Read the model definition and answer for the solid it produces. Units are mm, in the model's axes. A direction names the side the tool comes from. Give positions to 0.01 mm unless a question says otherwise; leave off trailing zeros. Order: outer loops, then holes, each group sorted by start corner. A loop starts at its lowest first (then second) coordinate and runs counter-clockwise, first axis right, second up.
```python
from build123d import *

# Parameters (mm, degrees)
F0_W     = 6.35
F0_H     = 6.35
F3_DEPTH = 61.214
F5_DEPTH = 6.35
F6_R     = 2.54


with BuildPart() as f1:
    # F0 (on Front) → F1 (revolve)
    with BuildSketch(Plane.XZ):
        with BuildLine():
            ThreePointArc((82.316182, 13.458223), (82.347533, 15.063283), (80.9625, 15.875))
            ThreePointArc((80.9625, 15.875), (69.73718, 11.22532), (65.0875, 0))
            Line((65.0875, 0), (71.4375, 8.40026))
            ThreePointArc((71.4375, 8.40026), (75.73724, 11.57526), (80.9625, 12.7))
            ThreePointArc((80.9625, 12.7), (81.738283, 12.902467), (82.316182, 13.458223))
        make_face()
        Polygon((71.4375, 8.40026), (65.0875, 0), (65.0875, -42.39974), (71.4375, -42.39974), (71.4375, -4.29974), align=None)
        with Locations((68.2625, -45.57474)):
            Rectangle(F0_W, F0_H)
        with BuildLine():
            Line((71.4375, -4.29974), (82.316182, 13.458223))
            ThreePointArc((82.316182, 13.458223), (81.738283, 12.902467), (80.9625, 12.7))
            ThreePointArc((80.9625, 12.7), (75.73724, 11.57526), (71.4375, 8.40026))
            Line((71.4375, 8.40026), (71.4375, -4.29974))
        make_face()
    revolve(axis=Axis((0, 0, -2.826434), (0, 0, -1)))

    # F2 (on face) → F3 (join)
    with BuildSketch(Plane(origin=(0, 0, -48.74974), x_dir=(1, 0, 0), z_dir=(0, 0, -1))):
        with BuildLine():
            ThreePointArc((-65.0875, -29.443739), (-69.831958, -15.060347), (-71.4375, 0))
            Line((-71.4375, 0), (-71.4375, -71.4375))
            Line((-71.4375, -71.4375), (0, -71.4375))
            ThreePointArc((0, -71.4375), (-15.060347, -69.831958), (-29.443739, -65.0875))
            Line((-29.443739, -65.0875), (-65.0875, -65.0875))
            Line((-65.0875, -65.0875), (-65.0875, -29.443739))
        make_face()
        with BuildLine():
            Line((71.4375, -71.4375), (71.4375, 0))
            ThreePointArc((71.4375, 0), (69.831958, -15.060347), (65.0875, -29.443739))
            Line((65.0875, -29.443739), (65.0875, -65.0875))
            Line((65.0875, -65.0875), (29.443739, -65.0875))
            ThreePointArc((29.443739, -65.0875), (15.060347, -69.831958), (0, -71.4375))
            Line((0, -71.4375), (71.4375, -71.4375))
        make_face()
    extrude(amount=-F3_DEPTH)

    # F4 (on face) → F5 (join)
    with BuildSketch(Plane(origin=(0, 0, -48.74974), x_dir=(1, 0, 0), z_dir=(0, 0, -1))):
        with BuildLine():
            ThreePointArc((3.175, -65.010015), (0, -65.0875), (-3.175, -65.010015))
            Line((-3.175, -65.010015), (-3.175, -71.4375))
            ThreePointArc((-3.175, -71.4375), (0, -71.508021), (3.175, -71.4375))
            Line((3.175, -71.4375), (3.175, -65.010015))
        make_face()
        with BuildLine():
            ThreePointArc((54.712824, 35.254638), (56.367428, 32.54375), (57.887824, 29.755377))
            Line((57.887824, 29.755377), (63.45419, 32.969119))
            ThreePointArc((63.45419, 32.969119), (61.927763, 35.75401), (60.27919, 38.468381))
            Line((60.27919, 38.468381), (54.712824, 35.254638))
        make_face()
        with BuildLine():
            ThreePointArc((-57.887824, 29.755377), (-56.367428, 32.54375), (-54.712824, 35.254638))
            Line((-54.712824, 35.254638), (-60.27919, 38.468381))
            ThreePointArc((-60.27919, 38.468381), (-61.927763, 35.75401), (-63.45419, 32.969119))
            Line((-63.45419, 32.969119), (-57.887824, 29.755377))
        make_face()
    extrude(amount=F5_DEPTH)

    # F6
    f6_edges = [f1.edges().sort_by_distance(p)[0] for p in [
        (57.496007, -36.861509, -55.09974),
        (60.671007, -31.362248, -55.09974),
        (-57.496007, -36.861509, -55.09974),
        (-60.671007, -31.362248, -55.09974),
        (3.175, 68.223757, -55.09974),
        (-3.175, 68.223757, -55.09974),
    ]]
    fillet(f6_edges, radius=F6_R)


solid = f1.part
```
1) Given pin 1 (10.5 mm diameter, centred on x = -45.5, z = -19.5, fed in from -Y); pin 2 (1.1 mm diameter, centred on y = 67.5, z = -51, fed in from -X) (3 decimals); pin 3 (2.5 mm diameter, centred on x = -61.5, y = -36, fed in from +Z); pin 4 (16 mm diameter, centred on x = 50.5, y = 60.5, fed in from +Z) (3 decimals), each flat-ended and moving along its own axis, determine where each tip first touches the part or whether it passes through.
Final values:
pin 1: stops at y = -59.02
pin 2: stops at x = -3.175
pin 3: stops at z = 13.44
pin 4: stops at z = 15.875
2) The part is cut by section B-B on z = 3. Determine the outline of the cut face in (x, y).
Final values:
outline: (-71.44, 25.67) arc R75.91 ccw (long way) to (71.44, 25.67) - (71.44, 71.44) - (25.67, 71.44) arc R75.91 ccw to (-25.67, 71.44) - (-71.44, 71.44) - close; hole circle Ø130.75 at (0, 0); hole (-65.09, 39.06) arc R75.91 cw to (-39.06, 65.09) - (-65.09, 65.09) - close; hole (39.06, 65.09) arc R75.91 cw to (65.09, 39.06) - (65.09, 65.09) - close
3) For a pull along X with two mould halves and no side action, classify faces 5 (the face through (48, 65.088, -19)), 6 (the face through (-3.175, 68, -51)), 7 (the face through (1.57, -71.42, -26.21)) as released by +X, released by -X, zero draft, split by the parting line, or undercut.
Final values:
face 5: undercut
face 6: released by -X
face 7: split by the parting line
4) The part is cut by section A-A on z = -30.5. Determine the outline of the cut face in (x, y) (1 decimal), and give its area (3 significant figures).
Final values:
outline: (-71.4, 0) arc R71.4 ccw to (71.4, 0) - (71.4, 71.4) - (-71.4, 71.4) - close; hole circle Ø130.2 at (0, 0); hole (-65.1, 29.4) arc R71.4 cw to (-29.4, 65.1) - (-65.1, 65.1) - close; hole (29.4, 65.1) arc R71.4 cw to (65.1, 29.4) - (65.1, 65.1) - close
area: 3,950 mm2
5) A tool of negligible diameter and unlimited length cuts with its end or side. For faces 1 (the face through (3.175, 68, -51)), 2 (the face through (-57.9, -36.3, -54.3)), 3 (the face through (56.345, -32.582, -51.88)), 4 (the face through (60.63, -31.34, -50.63)), from which of +Z, -Z, +X, -X, +Y, -Y can it reach the whole face along a straight path? Write none if from no direction.
Final values:
face 1: -Z, +X, +Y, -Y
face 2: -Z, -Y
face 3: +Z, -Z, +Y
face 4: -Z, +X, +Y
6) Consider L1, parallel to X at y = 0, z = -30; L2, parallel to Y at x = 41.5, z = -22; L3, parallel to Y at x = 38.5, z = -34.5. Determine where each line is inside the solid, lowest interval first.
Final values:
L1: x = -71.44 to -65.09, 65.09 to 71.44
L2: y = -58.15 to -50.14, 50.14 to 58.15, 65.09 to 71.44
L3: y = -60.18 to -52.48, 52.48 to 60.18, 65.09 to 71.44
7) The part is cut by section C-C on y = 57. Count the separate pieces of the cut face and the enclosed holes in it, and give its area (3 significant figures).
Final values:
separate pieces: 4
enclosed holes: 0
area: 2,460 mm2
